```python
from build123d import *

# Parameters (mm, degrees)
BOSS_EXTRUDE1_DEPTH = 2
BOSS_EXTRUDE4_DEPTH = 2
SKETCH6_R           = 3.25
SKETCH6_R_2         = 1.75
BOSS_EXTRUDE5_DEPTH = 6.5
BOSS_EXTRUDE2_START = -0.870835
SKETCH2_R           = 3.25
SKETCH2_R_2         = 1.75
BOSS_EXTRUDE2_DEPTH = 7.370835
BOSS_EXTRUDE3_START = -0.870835
SKETCH3_R           = 3.25
SKETCH3_R_2         = 1.75
BOSS_EXTRUDE3_DEPTH = 7.370835
SKETCH4_R           = 1.5
CUT_EXTRUDE1_DEPTH  = 2
CHAMFER1_SIZE       = 1


with BuildPart() as part:
    # Sketch1 → Boss-Extrude1 (new body)
    with BuildSketch(Plane(origin=(0, 0, 0), x_dir=(1, 0, 0), z_dir=(0, 1, 0))):
        with BuildLine():
            Line((-21.75, 3.25), (21.75, 3.25))
            ThreePointArc((21.75, 3.25), (25, 0), (21.75, -3.25))
            Line((21.75, -3.25), (-21.75, -3.25))
            ThreePointArc((-21.75, -3.25), (-25, 0), (-21.75, 3.25))
        make_face()
    extrude(amount=BOSS_EXTRUDE1_DEPTH)

    # Sketch5 → Boss-Extrude4 (add)
    with BuildSketch(Plane(origin=(0, 0, 0), x_dir=(1, 0, 0), z_dir=(0, 1, 0))):
        with BuildLine():
            Line((-3.25, 0), (3.25, 0))
            Line((3.25, 0), (3.25, 35))
            ThreePointArc((3.25, 35), (0, 38.25), (-3.25, 35))
            Line((-3.25, 35), (-3.25, 0))
        make_face()
    extrude(amount=BOSS_EXTRUDE4_DEPTH)

    # Sketch6 → Boss-Extrude5 (add)
    with BuildSketch(Plane(origin=(0, 2, 0), x_dir=(1, 0, 0), z_dir=(0, 1, 0))):
        with Locations(Location((0, 35, 0), (0, 0, 180))):
            Circle(SKETCH6_R)
        with Locations((0, 35)):
            Circle(SKETCH6_R_2, mode=Mode.SUBTRACT)
    extrude(amount=BOSS_EXTRUDE5_DEPTH)

    # Sketch2 → Boss-Extrude2 (add)
    with BuildSketch(Plane(origin=(-1.956973734, 7.303525404, 0), x_dir=(0, 0, -1), z_dir=(-0.25881904510252135, 0.9659258262890681, 0)).offset(BOSS_EXTRUDE2_START)):
        with Locations((0, 20.491248632)):
            Circle(SKETCH2_R)
        with Locations(Location((0, 20.491248632, 0), (0, 0, 270))):
            Circle(SKETCH2_R_2, mode=Mode.SUBTRACT)
    extrude(amount=BOSS_EXTRUDE2_DEPTH)

    # Sketch3 → Boss-Extrude3 (add)
    with BuildSketch(Plane(origin=(1.956973734, 7.303525404, 0), x_dir=(0, 0, -1), z_dir=(0.25881904510252135, 0.9659258262890681, 0)).offset(BOSS_EXTRUDE3_START)):
        with Locations((0, -20.491248632)):
            Circle(SKETCH3_R)
        with Locations(Location((0, -20.491248632, 0), (0, 0, 90))):
            Circle(SKETCH3_R_2, mode=Mode.SUBTRACT)
    extrude(amount=BOSS_EXTRUDE3_DEPTH)

    # Sketch4 → Cut-Extrude1 (cut)
    with BuildSketch(Plane(origin=(0, 2, 0), x_dir=(1, 0, 0), z_dir=(0, 1, 0))):
        with Locations(Location((-15, 0, 0), (0, 0, 270))):
            Circle(SKETCH4_R)
        with Locations(Location((15, 0, 0), (0, 0, 270))):
            Circle(SKETCH4_R)
    extrude(amount=-CUT_EXTRUDE1_DEPTH, mode=Mode.SUBTRACT)

    # Chamfer1
    chamfer1_edges = [part.edges().sort_by_distance(p)[0] for p in [
        (-15, 2, -1.5),
        (15, 2, -1.5),
    ]]
    chamfer(chamfer1_edges, length=CHAMFER1_SIZE)


solid = part.part
```
Build history of the part. All positions in model axes, mm. A direction names the side the tool comes from. Coordinates: 2 decimals unless noted, no trailing zeros. Write each loop counter-clockwise with the first axis right and the second up, starting at its lowest first coordinate (ties: lowest second). Pieces come first, ordered by that corner, then holes.
1. Band-saw the part on A-A, the plane x = 15. Give the cut face in (y, z).
Answer block:
outline: (0, -3.25) - (2, -3.25) - (2, -2.5) - (1, -1.5) - (0, -1.5) - close; (0, 1.5) - (1, 1.5) - (2, 2.5) - (2, 3.25) - (0, 3.25) - close
2. Band-saw the part on B-B, the plane z = 0. Give the number of separate pieces and of enclosed holes in the cut face, and give its area (3 significant figures).
Answer block:
separate pieces: 3
enclosed holes: 0
area: 125 mm2
3. Drill centre lines: probe 1 along X at (y, z) = (6.5, -35); probe 2 along X at (y, z) = (0.7, 0); probe 3 along Y at (x, z) = (-0.5, -6.5). Where is each one in solid material? Low to high.
Answer block:
probe 1: x = -3.25 to -1.75, 1.75 to 3.25
probe 2: x = -25 to -16.5, -13.5 to 13.5, 16.5 to 25
probe 3: y = 0 to 2
4. 3-axis set-ups, long thin cutter, end or side, ignore diameter. For faces 1 (the flat face through (-13, 1, -3.25)), 2 (the cylindrical face through (25, 1, 0)), 3 (the flat face through (3.25, 1, -19)), 4 (the cylindrical face through (-25, 1, 0)): which of +Z, -Z, +X, -X, +Y, -Y reach the whole face in a straight line?
Answer block:
face 1: -Z, -X, +Y, -Y
face 2: +X, -Y
face 3: -Z, +X, +Y, -Y
face 4: -X, -Y
5. Drop flat-ended pins along their axis: pin 1 (12 mm diameter, centred on x = -9, z = -19, fed in from -Y); pin 2 (2 mm diameter, centred on x = 0, z = -35.5, fed in from +Y); pin 3 (1 mm diameter, centred on x = 16.5, y = 1, fed in from -Z); pin 4 (3 mm diameter, centred on x = 0.5, z = -35, fed in from +Y). Give the stop position or say it passes through.
Answer block:
pin 1: stops at y = 0
pin 2: stops at y = 2
pin 3: stops at z = -3.25
pin 4: stops at y = 8.5
6. Pull direction X, two halves, no side cores. Call faces 5 (the flat face through (22, 2, 0)), 6 (the flat face through (-3.25, 1, -19)), 7 (the flat face through (12, 1, -3.25)): released by +X, released by -X, zero draft, split by the parting line, or undercut.
Answer block:
face 5: undercut
face 6: released by -X
face 7: zero draft
7. Band-saw the part on D-D, the plane x = 8. Give the cut face in (y, z).
Answer block:
outline: (0, -3.25) - (2, -3.25) - (2, 3.25) - (0, 3.25) - close
